from build123d import *

# Parameters (mm, degrees)
SKETCH_1_W      = 28
SKETCH_1_H      = 28
EXTRUDE_1_DEPTH = 38.5
SKETCH_2_R      = 11
EXTRUDE_2_DEPTH = 2
SKETCH_3_R      = 2.5
EXTRUDE_3_DEPTH = 13
CHAMFER_1_SIZE  = 3


with BuildPart() as part:
    # 草图1 → 凸台-拉伸1 (new body)
    with BuildSketch(Plane.XY):
        Rectangle(SKETCH_1_W, SKETCH_1_H)
    extrude(amount=EXTRUDE_1_DEPTH)

    # 草图2 → 凸台-拉伸2 (add)
    with BuildSketch(Plane.XY.offset(38.5)):
        Circle(SKETCH_2_R)
    extrude(amount=EXTRUDE_2_DEPTH)

    # 草图3 → 凸台-拉伸3 (add)
    with BuildSketch(Plane.XY.offset(40.5)):
        with Locations(Location((0, 0, 0), (0, 0, 180))):
            Circle(SKETCH_3_R)
    extrude(amount=EXTRUDE_3_DEPTH)

    # 倒角1
    chamfer_1_edges = [part.edges().sort_by_distance(p)[0] for p in [
        (14, -14, 19.25),
        (-14, -14, 19.25),
        (-14, 14, 19.25),
        (14, 14, 19.25),
    ]]
    chamfer(chamfer_1_edges, length=CHAMFER_1_SIZE)


solid = part.part
Source: CAD feature listing. Evaluate the final solid. Frame: model axes, mm. A direction names the side the tool comes from. Round coordinates to 2 decimals unless told otherwise and drop trailing zeros. Write each loop counter-clockwise with the first axis right and the second up, starting at its lowest first coordinate (ties: lowest second). Pieces come first, ordered by that corner, then holes. Notation, with made-up numbers: (19.5, 79) - (24.5, 79) arc R4 cw to (24.5, 86) - close; hole circle Ø2 at (-3.75, 81). An arc over 180 degrees is marked (long way). Use CSV: the item, a comma, the result in double quotes. Start each with the question number.
(1) Cut plane D-D, the plane x = 6.5. Return loops of the section in (y, z).
(2) Cut plane A-A, the plane y = 0. Return loops of the section in (x, z).
(3) Material intervals for probe 1 along Z at (x, y) = (8.25, 3); probe 2 along Z at (x, y) = (-12, 1.5); probe 3 along Y at (x, z) = (3, 39), sorted ascending. Write a range as [from, to].
(4) Set-up query: faces 1 (the face through (2.5, -0.1, 46.9)), 2 (the face through (0, 0, 0)). Return all of +Z, -Z, +X, -X, +Y, -Y with unobstructed straight access to the full face (end or side cutting, diameter ignored); none if empty.
(5) Cut plane C-C, the plane z = 5. Return loops of the section in (x, y), and give its area (3 significant figures).
(6) First-contact query: pin 1 Ø1 at (y, z) = (4.5, 47) entering from -X; pin 2 Ø2 at (x, y) = (-3.5, -0.5) entering from +Z. Flat tips, straight axial feed; report the tip coordinate or a pass-through.
Geometry says:
1,outline,"(-14, 0) - (14, 0) - (14, 38.5) - (8.87, 38.5) - (8.87, 40.5) - (-8.87, 40.5) - (-8.87, 38.5) - (-14, 38.5) - close"
2,outline,"(-14, 0) - (14, 0) - (14, 38.5) - (11, 38.5) - (11, 40.5) - (2.5, 40.5) - (2.5, 53.5) - (-2.5, 53.5) - (-2.5, 40.5) - (-11, 40.5) - (-11, 38.5) - (-14, 38.5) - close"
3,probe 1,"[0, 40.5]"
3,probe 2,"[0, 38.5]"
3,probe 3,"[-10.58, 10.58]"
4,face 1,"+Z"
4,face 2,"-Z, +X, -X, +Y, -Y"
5,outline,"(-14, -11) - (-11, -14) - (11, -14) - (14, -11) - (14, 11) - (11, 14) - (-11, 14) - (-14, 11) - close"
5,area,"766 mm²"
6,pin 1,"through"
6,pin 2,"z = 40.5"
